from build123d import *

# Parameters (mm, degrees)
F0_W     = 25.4
F0_H     = 25.4
F0_W_2   = 12.7
F0_H_2   = 12.7
F1_DEPTH = 25.4
F2_W     = 12.7
F2_H     = 12.7
F3_DEPTH = 43.942
F4_W     = 12.7
F4_H     = 12.7
F5_DEPTH = 39.116
F6_SIZE  = 2.54
F7_SIZE  = 2.54


with BuildPart() as f1:
    # F0 (on Top) → F1 (new body)
    with BuildSketch(Plane.XY):
        Rectangle(F0_W, F0_H)
        Rectangle(F0_W_2, F0_H_2, mode=Mode.SUBTRACT)
    extrude(amount=F1_DEPTH)

    # F2 (on Right) → F3 (cut, symmetric)
    with BuildSketch(Plane.YZ):
        with Locations((0, 12.7)):
            Rectangle(F2_W, F2_H)
    extrude(amount=F3_DEPTH, both=True, mode=Mode.SUBTRACT)

    # F4 (on Front) → F5 (cut, symmetric)
    with BuildSketch(Plane.XZ):
        with Locations((0, 12.7)):
            Rectangle(F4_W, F4_H)
    extrude(amount=F5_DEPTH, both=True, mode=Mode.SUBTRACT)

    # F6
    f6_edges = [f1.edges().sort_by_distance(p)[0] for p in [
        (0, -6.35, 0),
        (-6.35, 0, 0),
        (0, 6.35, 0),
        (6.35, 0, 0),
        (12.7, 6.35, 12.7),
        (12.7, 0, 19.05),
        (12.7, -6.35, 12.7),
        (12.7, 0, 6.35),
        (-12.7, -6.35, 12.7),
        (-12.7, 0, 19.05),
        (-12.7, 0, 6.35),
        (-12.7, 6.35, 12.7),
        (0, -6.35, 25.4),
        (-6.35, 0, 25.4),
        (0, 6.35, 25.4),
        (6.35, 0, 25.4),
        (6.35, 12.7, 12.7),
        (0, 12.7, 19.05),
        (0, 12.7, 6.35),
        (-6.35, 12.7, 12.7),
        (0, -12.7, 19.05),
        (6.35, -12.7, 12.7),
        (0, -12.7, 6.35),
        (-6.35, -12.7, 12.7),
    ]]
    chamfer(f6_edges, length=F6_SIZE)

    # F7
    f7_edges = [f1.edges().sort_by_distance(p)[0] for p in [
        (12.7, 0, 0),
        (12.7, -12.7, 12.7),
        (0, -12.7, 0),
        (0, -12.7, 25.4),
        (-12.7, -12.7, 12.7),
        (-12.7, 0, 0),
        (0, 12.7, 0),
        (12.7, 12.7, 12.7),
        (12.7, 0, 25.4),
        (0, 12.7, 25.4),
        (-12.7, 0, 25.4),
        (-12.7, 12.7, 12.7),
    ]]
    chamfer(f7_edges, length=F7_SIZE)


solid = f1.part
Verification items for the finished model (mm, model axes). A direction names the side the tool comes from. Coordinates: 2 decimals unless noted, no trailing zeros. Order: outer loops, then holes, each group sorted by start corner. A loop starts at its lowest first (then second) coordinate and runs counter-clockwise, first axis right, second up. Notation, with made-up numbers: M -25.75,77.25 L 19.25,77.25 A22 ccw 19.25,107.25 Z; hole C -30.5,33.25 d7. An arc over 180 degrees is marked long. Return JSON: item names as keys, results as strings.
1) Thickness scan on L1, parallel to Y at x = -10, z = 18.5; L2, parallel to X at y = 8.5, z = 11.75. Record the ranges inside material, lowest first. Write a range as [from, to].
Answer list:
{"L1": "[-12.7, -6.35], [6.35, 12.7]", "L2": "[-12.31, -6.35], [6.35, 12.31]"}
2) Cross-section at C-C, the plane x = 3.25. Record the boundary of the cut face in (y, z).
Answer list:
{"outline": "M -12.7,2.54 L -10.16,0 L -8.89,0 L -6.35,2.54 L -6.35,6.35 L -10.16,6.35 L -12.7,3.81 Z; M -12.7,21.59 L -10.16,19.05 L -6.35,19.05 L -6.35,22.86 L -8.89,25.4 L -10.16,25.4 L -12.7,22.86 Z; M 6.35,2.54 L 8.89,0 L 10.16,0 L 12.7,2.54 L 12.7,3.81 L 10.16,6.35 L 6.35,6.35 Z; M 6.35,19.05 L 10.16,19.05 L 12.7,21.59 L 12.7,22.86 L 10.16,25.4 L 8.89,25.4 L 6.35,22.86 Z"}
3) Access from +Z, -Z, +X, -X, +Y, -Y to the whole of each face (thin tool, end or side, straight path). Record for faces 1 (the flat face through (0.12, -11.41, 20.3)), 2 (the flat face through (-7.6, 11.41, 12.82)), 3 (the flat face through (-11.41, 0.12, 5.1)), 4 (the flat face through (8, 0, 6.35)).
Answer list:
{"face 1": "-Y", "face 2": "+Y", "face 3": "-X", "face 4": "+X, -X"}
4) Cross-section at A-A, the plane z = 3. Record the boundary of the cut face in (x, y).
Answer list:
{"outline": "M -12.7,-10.16 L -10.16,-12.7 L 10.16,-12.7 L 12.7,-10.16 L 12.7,10.16 L 10.16,12.7 L -10.16,12.7 L -12.7,10.16 Z; hole M -6.35,-6.35 L 6.35,-6.35 L 6.35,6.35 L -6.35,6.35 Z"}
5) Cross-section at B-B, the plane y = -9.25. Record the boundary of the cut face in (x, z), and give its area (3 significant figures).
Answer list:
{"outline": "M -12.7,2.54 L -10.16,0 L 10.16,0 L 12.7,2.54 L 12.7,22.86 L 10.16,25.4 L -10.16,25.4 L -12.7,22.86 Z; hole M -6.35,6.35 L 6.35,6.35 L 6.35,19.05 L -6.35,19.05 Z", "area": "471 mm2"}
6) Release check for a two-part mould opening along Y. For faces 5 (the flat face through (-8, 6.35, 13)), 6 (the flat face through (-9.1, 12.7, 12.7)), 7 (the flat face through (0, -8, 6.35)) record: +Y half, -Y half, draft (parallel to the pull), parting line (faces both ways), or undercut.
Answer list:
{"face 5": "undercut", "face 6": "+Y half", "face 7": "draft"}
7) Gauge pin test, flat ends, axial feed: pin 1 (1.5 mm diameter, centred on x = 7.5, y = 7.5, fed in from -Z); pin 2 (1.9 mm diameter, centred on y = -2.5, z = 5, fed in from +X); pin 3 (4 mm diameter, centred on y = -6.5, z = 10, fed in from +X); pin 4 (5 mm diameter, centred on x = -2.5, y = 3.5, fed in from +Z). Record the tip position at first contact, or that the pin passes through.
Answer list:
{"pin 1": "z = 0.64", "pin 2": "x = 12.46", "pin 3": "x = 12.31", "pin 4": "through"}
